Check sheet for the drawn part. Datum: minimum x, y, z corner. Units: mm. Round coordinates to 2 decimals unless told otherwise and drop trailing zeros. Order: outer loops, then holes, each group sorted by start corner. A loop starts at its lowest first (then second) coordinate and runs counter-clockwise, first axis right, second up. Notation, with made-up numbers: (-16.75, 49) -> (26.25, 49) arc R7 cw to (26.25, 61) -> close; hole circle Ø3 at (-2.5, 13.25). An arc over 180 degrees is marked (long way). Write item = value, one per line. Start each with the question number.
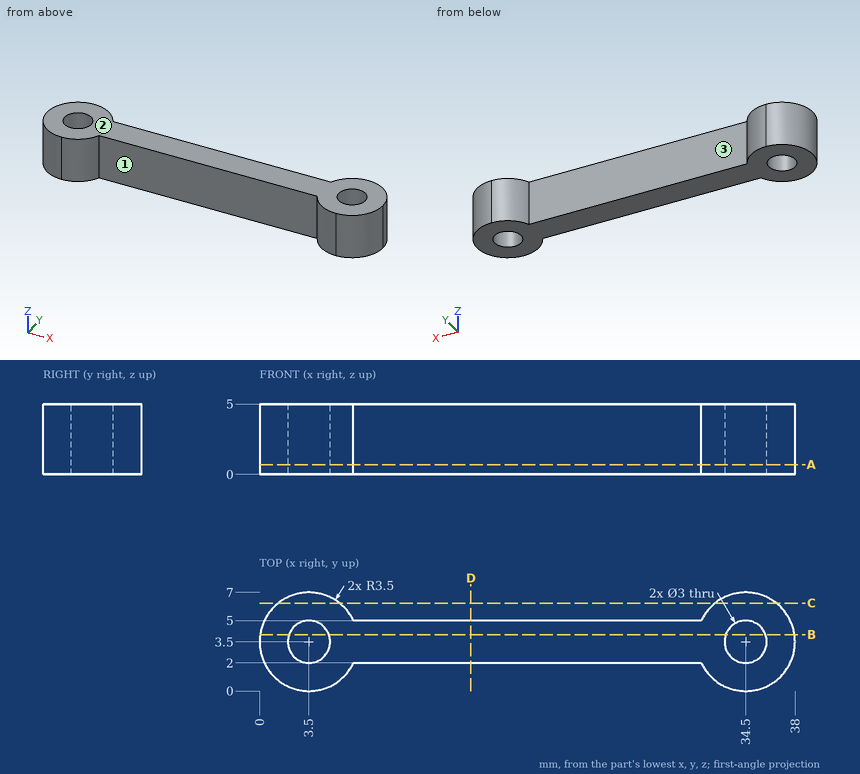
(1) Cross-section at D-D (x = 15). Enter the section's corners in (y, z), and give its area (3 significant figures).
(2) Cross-section at C-C (y = 6.25). Enter the section's corners in (x, z).
(3) Scan lines: line 1 along Y through (x, z) = (34.5, 3.8); line 2 along X through (y, z) = (2.5, 3.4); line 3 along Y through (x, z) = (29, 3.25). Record each from-to range of solid material in increasing order. Write a range as from..to.
(4) Depth check by flat-ended pin: pin 1 (4 mm diameter, centred on x = 8, y = 3, fed in from -Z); pin 2 (1.5 mm diameter, centred on x = 18.5, z = 2.5, fed in from -Y); pin 3 (3 mm diameter, centred on x = 21, z = 3.5, fed in from +Y). Enter the tip coordinate at first touch or a pass-through.
(5) Draft check along X on the marked faces 1, 2 and 3. Enter one of: +X half, -X half, draft (parallel to the pull), parting line (faces both ways), or undercut.
(6) Cross-section at A-A (z = 0.7). Enter the section's corners in (x, y).
(7) Cross-section at B-B (y = 4). Enter the section's corners in (x, z), and give its area (3 significant figures).
Outcome:
q1.outline = (2, 0) -> (5, 0) -> (5, 5) -> (2, 5) -> close
q1.area = 15.0 mm^2
q2.outline = (1.33, 0) -> (5.67, 0) -> (5.67, 5) -> (1.33, 5) -> close; (32.33, 0) -> (36.67, 0) -> (36.67, 5) -> (32.33, 5) -> close
q3.line_1 = 0..2, 5..7
q3.line_2 = 0.15..2.38, 4.62..33.38, 35.62..37.85
q3.line_3 = 2..5
q4.pin_1 = 0
q4.pin_2 = 2
q4.pin_3 = 5
q5.face_1 = undercut
q5.face_2 = draft
q5.face_3 = undercut
q6.outline = (6.66, 2) -> (31.34, 2) arc R3.5 ccw (long way) to (31.34, 5) -> (6.66, 5) arc R3.5 ccw (long way) to start; hole circle Ø3 at (3.5, 3.5); hole circle Ø3 at (34.5, 3.5)
q7.outline = (0.04, 0) -> (2.09, 0) -> (2.09, 5) -> (0.04, 5) -> close; (4.91, 0) -> (33.09, 0) -> (33.09, 5) -> (4.91, 5) -> close; (35.91, 0) -> (37.96, 0) -> (37.96, 5) -> (35.91, 5) -> close
q7.area = 161 mm^2
